Here's the drawing with two shaded views (mm, measured from the low corner). I have some questions. A direction names the side the tool comes from. Round coordinates to 2 decimals unless told otherwise and drop trailing zeros. Order: outer loops, then holes, each group sorted by start corner. A loop starts at its lowest first (then second) coordinate and runs counter-clockwise, first axis right, second up.
Q1. If we section it at C-C (x = 110): Please give me the cut outline in (y, z), plus the area to 3 significant figures.
Q2. If we section it at A-A (y = 63.5): Please give me the cut outline in (x, z).
Q3. For the marked faces 1, 2 and 3, which set-ups out of +Z, -Z, +X, -X, +Y, -Y let a thin tool reach every point of the face, with its end or its side?
Q4. Will these pins go through, and if not, where does the flat tip stop? P1, Ø3, axis at y = 64, z = 36.5, coming from the -X side; P2, Ø8, axis at x = 15.5, z = 54.5, coming from the +Y side; P3, Ø1.5, axis at x = 118.5, y = 74, coming from the -Z side.
Q5. If we section it at B-B (z = 74): Please give me the cut outline in (x, y), plus the area to 3 significant figures.
Q6. If I drill on line 1 (Z direction, x = 61.5, y = 64); line 2 (X direction, y = 54.5, z = 78.5), over which ranges is the centre line in solid material (lowest first)?
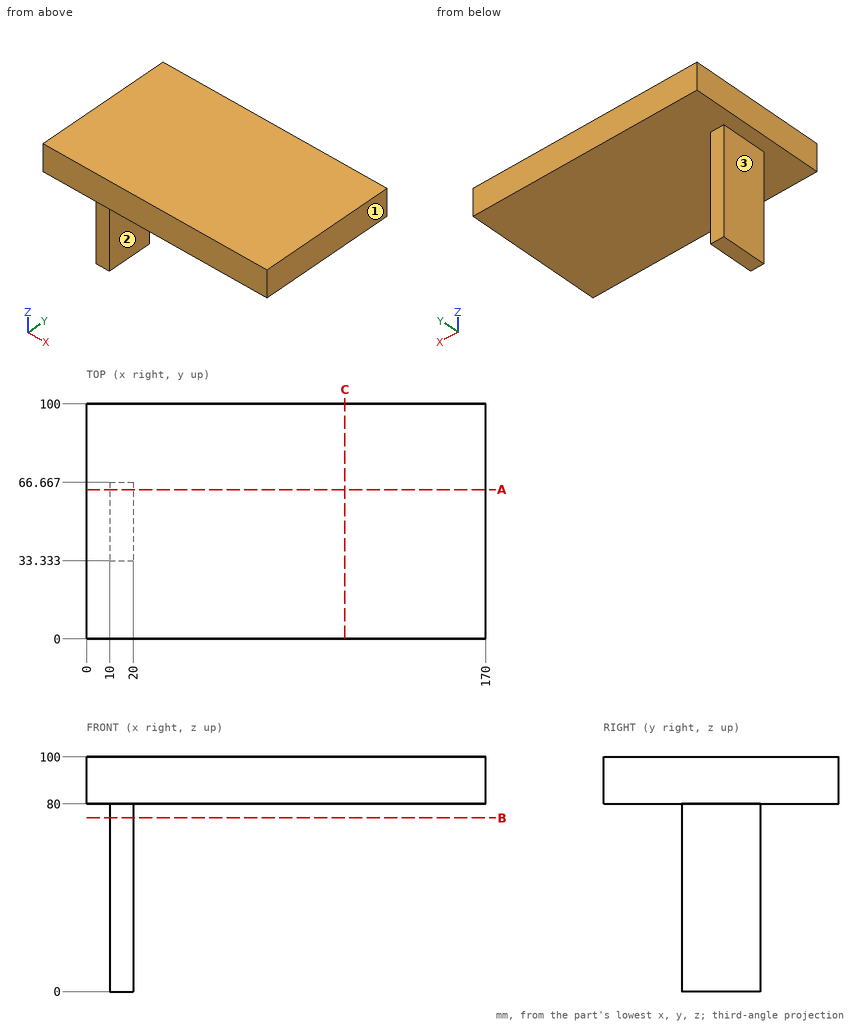
Solution:
1. outline: (0, 80) - (100, 80) - (100, 100) - (0, 100) - close
1. area: 2,000 mm2
2. outline: (0, 80) - (10, 80) - (10, 0) - (20, 0) - (20, 80) - (170, 80) - (170, 100) - (0, 100) - close
3. face 1: +Z, -Z, +X, +Y, -Y
3. face 2: -Z, +X, +Y, -Y
3. face 3: -Z, -X, +Y, -Y
4. P1: stops at x = 10
4. P2: stops at y = 66.67
4. P3: stops at z = 80
5. outline: (10, 33.33) - (20, 33.33) - (20, 66.67) - (10, 66.67) - close
5. area: 333 mm2
6. line 1: z = 80 to 100
6. line 2: x = 10 to 20
